Here's the drawing with two shaded views (mm, measured from the low corner). I have some questions. Round coordinates to 2 decimals unless told otherwise and drop trailing zeros. Loops run counter-clockwise (first coordinate to the right, second up) from the corner with the lowest first, then second, coordinate; pieces in that order, holes last. Notation, with made-up numbers: (56, 2.25) - (78, 2.25) arc R19 cw to (78, 12.25) - close; hole circle Ø9 at (-27.5, -6.5). An arc over 180 degrees is marked (long way). Answer as CSV lines item,"result".
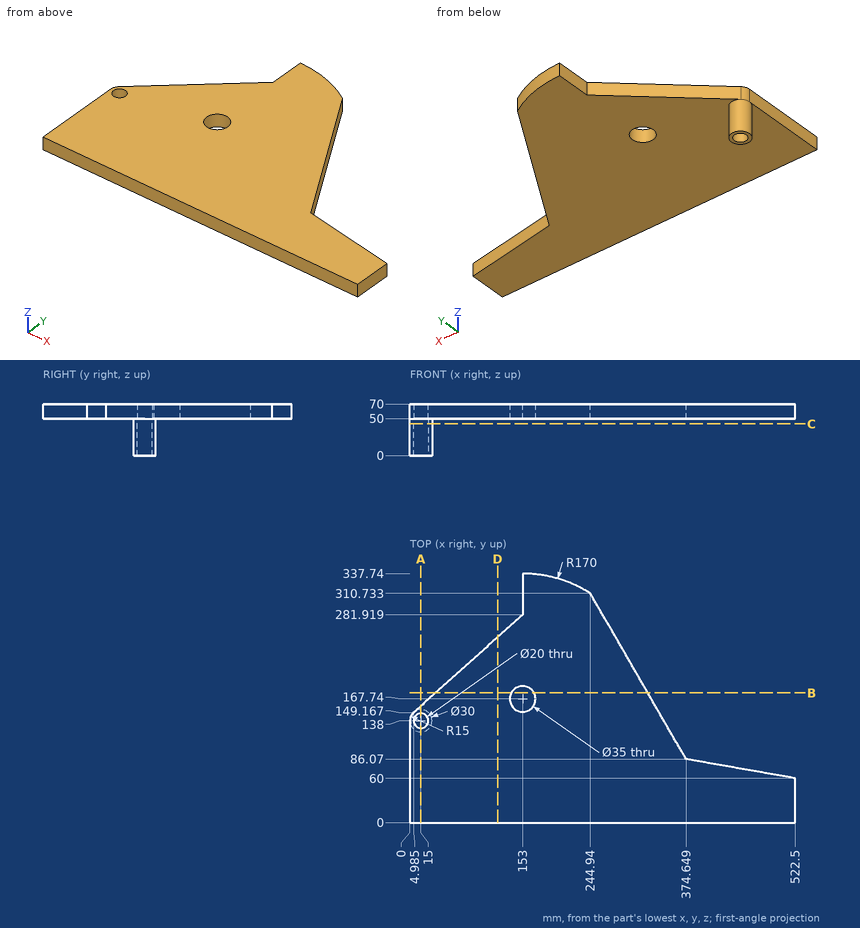
Q1. If I drill on line 1 along Y through (x, z) = (15, 35); line 2 along X through (y, z) = (136.5, 41) (1 decimal); line 3 along Z through (x, y) = (224.5, 67), over which ranges is the centre line in solid material (lowest first)? Write a range as [from, to].
Checks:
line 1,"[123, 128], [148, 153]"
line 2,"[0.1, 5.1], [24.9, 29.9]"
line 3,"[50, 70]"
Q2. Imagine slicing it at B-B (y = 176). Write out the boundary of the cut face in (x, z), then the cut area to 3 significant figures.
Checks:
outline,"(34.9, 50) - (137.57, 50) - (137.57, 70) - (34.9, 70) - close; (168.43, 50) - (322.73, 50) - (322.73, 70) - (168.43, 70) - close"
area,"5,140 mm²"
Q3. Imagine slicing it at A-A (x = 15). Write out the boundary of the cut face in (y, z), then the cut area to 3 significant figures.
Checks:
outline,"(0, 50) - (123, 50) - (123, 0) - (128, 0) - (128, 70) - (0, 70) - close; (148, 0) - (153, 0) - (153, 50) - (158.15, 50) - (158.15, 70) - (148, 70) - close"
area,"3,260 mm²"
Q4. I'm going to push flat-ended pins straight in: pin 1 Ø10 at (y, z) = (321, 60) entering from -X; pin 2 Ø5 at (y, z) = (225, 57) entering from -X; pin 3 Ø8 at (y, z) = (146, 58.5) entering from -X. Where does each tip first touch, or does it pass through?
Checks:
pin 1,"x = 153"
pin 2,"x = 86.75"
pin 3,"x = 0.54"
Q5. Imagine slicing it at D-D (x = 119). Write out the boundary of the cut face in (y, z) (1 decimal).
Checks:
outline,"(0, 50) - (251.4, 50) - (251.4, 70) - (0, 70) - close"
Q6. Imagine slicing it at C-C (z = 43). Write out the boundary of the cut face in (x, y).
Checks:
outline,"circle Ø30 at (15, 138); hole circle Ø20 at (15, 138)"
